Autodesk Inventor part; units mm, degrees
ref_plane "YZ Plane" through (0, 0, 0) normal (1, 0, 0) x (0, 1, 0)
ref_plane "XZ Plane" through (0, 0, 0) normal (0, 1, 0) x (-1, 0, 0)
ref_plane "XY Plane" through (0, 0, 0) normal (0, 0, 1) x (1, 0, 0)
sketch "Sketch1" plane through (0, 0, 0) normal (0, 0, 1) x (1, 0, 0)
  line L0 (-25, 5) -> (25, 5)
  line L1 (25, 5) -> (25, -5)
  line L2 (25, -5) -> (-25, -5)
  line L3 (-25, -5) -> (-25, 5)
  line L4 (-25, 5) -> (25, -5) construction
  line L5 (25, 5) -> (-25, -5) construction
  circle A0 centre (-20, 0) radius 1.75
  line L6 (0, 0) -> (0, -5.5046) construction
  circle A1 centre (20, 0) radius 1.75
  dimension "d0" = 50
  dimension "d1" = 10
  dimension "d2" = 3.5
  dimension "d3" = 40
  dimension "d4" = 5
extrude "Plate1" add sketch "Sketch1" along normal blind 1
sketch "Sketch2" plane through (-25, 6, 2) normal (0, 1, 0) x (-1, 0, 0)
  line L0 (-50, 0) -> (0, 0)
  line L1 (0, 0) -> (0, 10)
  line L2 (0, 10) -> (-50, 10)
  line L3 (-50, 10) -> (-50, 0)
edge flange "Flange1" height 12 angle 90 thickness 1 bend radius 1 thickness toward (0, 1, 0) relief tear relief width 1 relief depth 0.5 edges at (0, 5, 1) wall of the first edge with corners at (25, 6, 2) (-25, 6, 2) (-25, 6, 12) (25, 6, 12)
bend "Bend1"
corner "Corner1"
sketch "Sketch3" plane through (-25, 6, 12) normal (0, -1, 0) x (1, 0, 0)
  circle A0 centre (41, -5) radius 2.25
  circle A1 centre (9, -5) radius 2.25
  line L0 (25, -12) -> (25, 5.1941) construction
  line L1 (50, -11) -> (0, -11) construction
  dimension "d20" = 4.5
  dimension "d21" = 4.5
  dimension "d22" = 32
  dimension "d23" = 6
extrude "Cut1" cut sketch "Sketch3" against normal blind 1
sketch "Sketch4" plane through (-25, 7, 12) normal (0, 1, 0) x (1, 0, 0)
  line L0 (50, 0) -> (0, 0)
  line L1 (35, 10) -> (15, 10)
  line L2 (15, 10) -> (15, 0)
  line L3 (15, 0) -> (35, 0)
  line L4 (35, 0) -> (35, 10)
  line L5 (35, 10) -> (15, 0) construction
  line L6 (15, 10) -> (35, 0) construction
  line L7 (50, 10) -> (0, 10)
  point P0 (25, 12)
  point P1 (25, 5)
  dimension "d26" = 20
extrude "Cut2" cut sketch "Sketch4" against normal blind 1
equation "\"d20\" = d21"
equation "\"d24\" = 厚度"
equation "\"d27\" = 厚度"
equation "\"d9\" = 厚度"
equation "\"d10\" = 折彎離隙寬度"
equation "\"d11\" = 折彎離隙深度"
equation "\"d12\" = 最小剩餘"
equation "\"d13\" = 轉移半徑"
equation "\"d16\" = 折彎半徑"
equation "\"d17\" = 轉角離隙大小"
equation "\"d18\" = 間隙大小"
equation "\"d19\" = Jacobi半徑大小"
equation "\"折彎半徑\" = 厚度"
equation "\"折彎離隙寬度\" = 厚度"
equation "\"折彎離隙深度\" = 0.5 * 厚度"
equation "\"轉角離隙大小\" = 4 * 厚度"
equation "\"最小剩餘\" = 2 * 厚度"
equation "\"轉移半徑\" = 折彎半徑"
equation "\"Jacobi半徑大小\" = 折彎半徑"
equation "\"間隙大小\" = 厚度"
properties part number "fan_fix_plate_connect2"
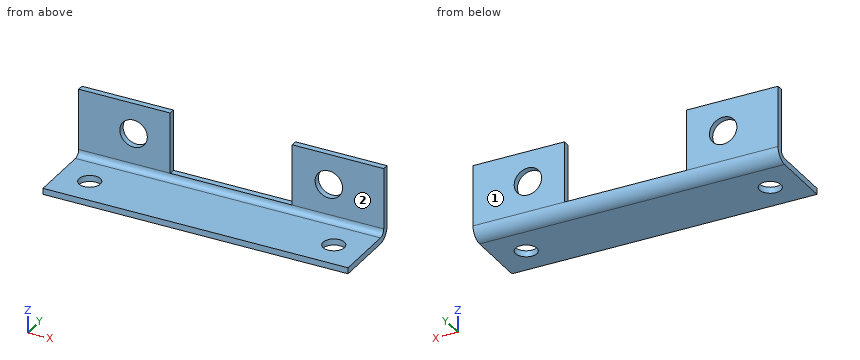
The model under review builds one solid part; all positions refer to its coordinate system, in mm. Face numbers are marked on the shaded views. A direction names the side the tool comes from. Round coordinates to 2 decimals unless told otherwise and drop trailing zeros. Order: outer loops, then holes, each group sorted by start corner. A loop starts at its lowest first (then second) coordinate and runs counter-clockwise, first axis right, second up. Notation, with made-up numbers: (62.5, 53) - (90.5, 53) arc R16 cw to (90.5, 61) - close; hole circle Ø4 at (47.25, -31). An arc over 180 degrees is marked (long way). Answer in a Markdown table with one row per item.
(1) Take a section at B-B on x = 20. Write out the cut boundary in (y, z), plus the area to 3 significant figures.
Result set:
| item | result |
|---|---|
| outline | (-5, 0) - (-1.75, 0) - (-1.75, 1) - (-5, 1) - close; (1.75, 0) - (5, 0) arc R2 ccw to (7, 2) - (7, 12) - (6, 12) - (6, 2) arc R1 cw to (5, 1) - (1.75, 1) - close |
| area | 18.9 mm2 |
(2) Take a section at D-D on y = -1. Write out the cut boundary in (x, z).
Result set:
| item | result |
|---|---|
| outline | (-25, 0) - (-21.44, 0) - (-21.44, 1) - (-25, 1) - close; (-18.56, 0) - (18.56, 0) - (18.56, 1) - (-18.56, 1) - close; (21.44, 0) - (25, 0) - (25, 1) - (21.44, 1) - close |
(3) For line 1 (Z direction, x = -16.5, y = -0.75); line 2 (Y direction, x = -11, z = 7.75); line 3 (Y direction, x = -21.5, z = 0.75), list the stretches that pass through material, from the lowest coordinate up. Write a range as from..to.
Result set:
| item | result |
|---|---|
| line 1 | z = 0..1 |
| line 2 | y = 6..7 |
| line 3 | y = -5..-0.9, 0.9..6.56 |
(4) Take a section at A-A on z = 3. Write out the cut boundary in (x, y), plus the area to 3 significant figures.
Result set:
| item | result |
|---|---|
| outline | (-25, 6) - (-10, 6) - (-10, 7) - (-25, 7) - close; (10, 6) - (25, 6) - (25, 7) - (10, 7) - close |
| area | 30.0 mm2 |
(5) Take a section at C-C on z = 7. Write out the cut boundary in (x, y).
Result set:
| item | result |
|---|---|
| outline | (-25, 6) - (-18.25, 6) - (-18.25, 7) - (-25, 7) - close; (-13.75, 6) - (-10, 6) - (-10, 7) - (-13.75, 7) - close; (10, 6) - (13.75, 6) - (13.75, 7) - (10, 7) - close; (18.25, 6) - (25, 6) - (25, 7) - (18.25, 7) - close |
(6) Clearance check with flat-ended pins moving along their axes: P1, Ø5, axis at x = -9.5, y = -2, coming from the +Z side; P2, Ø4, axis at x = 16, z = 7, coming from the -Y side. State where each tip first meets the part, or that it passes through.
Result set:
| item | result |
|---|---|
| P1 | stops at z = 1 |
| P2 | passes through |
(7) Machinability: for the marked faces 1 and 2, which of the approach directions +Z, -Z, +X, -X, +Y, -Y give a long, thin tool a straight path to every point of the face, cutting with its end or side? Answer none if there is none.
Result set:
| item | result |
|---|---|
| face 1 | +Z, -Z, +X, -X, +Y |
| face 2 | +Z, +X, -X, -Y |
